from build123d import *

# Parameters (mm, degrees)
CROQUIS1_W              = 50
CROQUIS1_H              = 66
CROQUIS1_W_2            = 43
CROQUIS1_H_2            = 30
SALIENTE_EXTRUIR1_DEPTH = 15
CROQUIS2_R              = 1.5
CROQUIS2_W              = 12
CROQUIS2_H              = 10
CORTAR_EXTRUIR5_DEPTH   = 67
CROQUIS3_W              = 10.5
CROQUIS3_H              = 2
CORTAR_EXTRUIR2_DEPTH   = 12
CROQUIS5_W              = 10.5
CROQUIS5_H              = 2
CORTAR_EXTRUIR3_DEPTH   = 12


with BuildPart() as part:
    # Croquis1 → Saliente-Extruir1 (new body)
    with BuildSketch(Plane.XY):
        with Locations((25, 33)):
            Rectangle(CROQUIS1_W, CROQUIS1_H)
        with Locations((23.5, 33)):
            Rectangle(CROQUIS1_W_2, CROQUIS1_H_2, mode=Mode.SUBTRACT)
    extrude(amount=SALIENTE_EXTRUIR1_DEPTH)

    # Croquis2 → Cortar-Extruir5 (cut, through all)
    with BuildSketch(Plane.XZ):
        with Locations(Location((42, 7.5, 0), (0, 0, 270))):  # turned: the seam where the file's is
            Circle(CROQUIS2_R)
        with Locations(Location((8, 7.5, 0), (0, 0, 270))):  # turned: the seam where the file's is
            Circle(CROQUIS2_R)
        with Locations((25, 5)):
            Rectangle(CROQUIS2_W, CROQUIS2_H)
    extrude(amount=-CORTAR_EXTRUIR5_DEPTH, mode=Mode.SUBTRACT)

    # Croquis3 → Cortar-Extruir2 (cut)
    with BuildSketch(Plane.ZY):
        with Locations((5.25, 61)):
            Rectangle(CROQUIS3_W, CROQUIS3_H)
        with Locations((5.25, 5)):
            Rectangle(CROQUIS3_W, CROQUIS3_H)
    extrude(amount=-CORTAR_EXTRUIR2_DEPTH, mode=Mode.SUBTRACT)

    # Croquis5 → Cortar-Extruir3 (cut)
    with BuildSketch(Plane(origin=(50, 0, 0), x_dir=(0, 0, -1), z_dir=(1, 0, 0))):
        with Locations((-5.25, 5)):
            Rectangle(CROQUIS5_W, CROQUIS5_H)
        with Locations((-5.25, 61)):
            Rectangle(CROQUIS5_W, CROQUIS5_H)
    extrude(amount=-CORTAR_EXTRUIR3_DEPTH, mode=Mode.SUBTRACT)


solid = part.part
Build history of the part. All positions in model axes, mm. A direction names the side the tool comes from. Give positions to 0.01 mm unless a question says otherwise; leave off trailing zeros. Order: outer loops, then holes, each group sorted by start corner. A loop starts at its lowest first (then second) coordinate and runs counter-clockwise, first axis right, second up. Notation, with made-up numbers: M -21.5,75 L 30.5,75 A11 ccw 30.5,93 Z; hole C 73.5,88.5 d7. An arc over 180 degrees is marked long. Put each result on its own line as item: value.
Item 1: Cut at A-A on x = 22. Write the cut outline in (y, z), then the cut area to 3 significant figures.
Results are:
outline: M 0,10 L 18,10 L 18,15 L 0,15 Z; M 48,10 L 66,10 L 66,15 L 48,15 Z
area: 180 mm2
Item 2: Cut at C-C on y = 44. Write the cut outline in (x, z).
Results are:
outline: M 0,0 L 2,0 L 2,15 L 0,15 Z; M 45,0 L 50,0 L 50,15 L 45,15 Z
Item 3: Wall check: probe 1 along Y at (x, z) = (8, 1.75); probe 2 along X at (y, z) = (13.5, 7.5); probe 3 along Y at (x, z) = (47, 1.25). Give the ranges that are in metal, low to high.
Results are:
probe 1: 0 to 4, 6 to 18, 48 to 60, 62 to 66
probe 2: 0 to 6.5, 9.5 to 19, 31 to 40.5, 43.5 to 50
probe 3: 0 to 4, 6 to 60, 62 to 66
Item 4: Which spindle directions (+Z, -Z, +X, -X, +Y, -Y) get a long thin tool onto all of the face, cutting with end or side? Do faces 1 (the face through (19, 9, 5)), 2 (the face through (44, 6, 5)), 3 (the face through (23, 48, 11)). Say none if no direction does.
Results are:
face 1: -Z, +Y, -Y
face 2: -Z, +X
face 3: +Z, -Z
Item 5: Pull direction X, two halves, no side cores. Call faces 4 (the face through (12, 5, 5)), 5 (the face through (44, 61, 10.5)), 6 (the face through (45, 33, 7)): +X half, -X half, draft (parallel to the pull), parting line (faces both ways), or undercut.
Results are:
face 4: -X half
face 5: draft
face 6: undercut
Item 6: Cut at D-D on x = 42. Count the separate pieces of the cut face and the enclosed holes in it, then the cut area to 3 significant figures.
Results are:
separate pieces: 6
enclosed holes: 0
area: 402 mm2
Item 7: Drop flat-ended pins along their axis: pin 1 Ø2.5 at (x, z) = (42, 7.5) entering from +Y; pin 2 Ø3.5 at (x, y) = (24.5, 5) entering from -Z; pin 3 Ø1 at (x, y) = (7, 61) entering from -Z; pin 4 Ø0.6 at (y, z) = (60.5, 4) entering from -X. Give the stop position or say it passes through.
Results are:
pin 1: through
pin 2: z = 10
pin 3: z = 10.5
pin 4: x = 12
